Check sheet for the modelled part. Datum: model origin and axes. Units: mm. A direction names the side the tool comes from. Round coordinates to 2 decimals unless told otherwise and drop trailing zeros. Loops run counter-clockwise (first coordinate to the right, second up) from the corner with the lowest first, then second, coordinate; pieces in that order, holes last. Notation, with made-up numbers: (4, 84.5) -> (25, 84.5) arc R14 ccw to (25, 109.5) -> close; hole circle Ø11 at (1.25, 4). An arc over 180 degrees is marked (long way). Return JSON: item names as keys, results as strings.
Autodesk Inventor part; units mm, degrees
ref_plane "YZ Plane" through (0, 0, 0) normal (1, 0, 0) x (0, 1, 0)
ref_plane "XZ Plane" through (0, 0, 0) normal (0, 1, 0) x (-1, 0, 0)
ref_plane "XY Plane" through (0, 0, 0) normal (0, 0, 1) x (1, 0, 0)
sketch "Sketch5" plane through (0, 0, 0) normal (0, 1, 0) x (-1, 0, 0)
  circle A0 centre (177.8, -63.5) radius 3.9688
  circle A1 centre (50.8, -63.5) radius 3.9687
  line L0 (6.35, 0) -> (6.35, -6.35)
  line L1 (6.35, -6.35) -> (0, -6.35)
  line L2 (0, -6.35) -> (0, -12.7)
  line L3 (0, -12.7) -> (6.35, -12.7)
  line L4 (6.35, -12.7) -> (6.35, -19.05)
  line L5 (6.35, -19.05) -> (0, -19.05)
  line L6 (0, -19.05) -> (0, -25.4)
  line L7 (0, -25.4) -> (6.35, -25.4)
  line L8 (6.35, -25.4) -> (6.35, -31.75)
  line L9 (6.35, -31.75) -> (0, -31.75)
  line L10 (0, -31.75) -> (0, -38.1)
  line L11 (0, -38.1) -> (6.35, -38.1)
  line L12 (6.35, -38.1) -> (6.35, -44.45)
  line L13 (6.35, -44.45) -> (0, -44.45)
  line L14 (0, -44.45) -> (0, -50.8)
  line L15 (0, -50.8) -> (6.35, -50.8)
  line L16 (6.35, -50.8) -> (6.35, -57.15)
  line L17 (6.35, -57.15) -> (0, -57.15)
  line L18 (0, -57.15) -> (0, -63.5)
  line L19 (0, -63.5) -> (6.35, -63.5)
  line L20 (6.35, -63.5) -> (6.35, -69.85)
  line L21 (6.35, -69.85) -> (0, -69.85)
  line L22 (0, -69.85) -> (0, -76.2)
  line L23 (0, -76.2) -> (6.35, -76.2)
  line L24 (6.35, -76.2) -> (6.35, -82.55)
  line L25 (6.35, -82.55) -> (0, -82.55)
  line L26 (0, -82.55) -> (0, -88.9)
  line L27 (0, -88.9) -> (6.35, -88.9)
  line L28 (6.35, -88.9) -> (6.35, -95.25)
  line L29 (6.35, -95.25) -> (0, -95.25)
  line L30 (0, -95.25) -> (0, -101.6)
  line L31 (0, -101.6) -> (6.35, -101.6)
  line L32 (6.35, -101.6) -> (6.35, -107.95)
  line L33 (6.35, -107.95) -> (0, -107.95)
  line L34 (0, -107.95) -> (0, -114.3)
  line L35 (0, -114.3) -> (6.35, -114.3)
  line L36 (6.35, -114.3) -> (6.35, -120.65)
  line L37 (6.35, -120.65) -> (0, -120.65)
  line L38 (0, -120.65) -> (0, -127)
  line L39 (0, -127) -> (6.35, -127)
  line L40 (6.35, -127) -> (6.35, -133.35)
  line L41 (222.25, -133.35) -> (222.25, -127)
  line L42 (222.25, -127) -> (228.6, -127)
  line L43 (228.6, -127) -> (228.6, -120.65)
  line L44 (228.6, -120.65) -> (222.25, -120.65)
  line L45 (222.25, -120.65) -> (222.25, -114.3)
  line L46 (222.25, -114.3) -> (228.6, -114.3)
  line L47 (228.6, -114.3) -> (228.6, -107.95)
  line L48 (228.6, -107.95) -> (222.25, -107.95)
  line L49 (222.25, -107.95) -> (222.25, -101.6)
  line L50 (222.25, -101.6) -> (228.6, -101.6)
  line L51 (228.6, -101.6) -> (228.6, -95.25)
  line L52 (228.6, -95.25) -> (222.25, -95.25)
  line L53 (222.25, -95.25) -> (222.25, -88.9)
  line L54 (222.25, -88.9) -> (228.6, -88.9)
  line L55 (228.6, -88.9) -> (228.6, -82.55)
  line L56 (228.6, -82.55) -> (222.25, -82.55)
  line L57 (222.25, -82.55) -> (222.25, -76.2)
  line L58 (222.25, -76.2) -> (228.6, -76.2)
  line L59 (228.6, -76.2) -> (228.6, -69.85)
  line L60 (228.6, -69.85) -> (222.25, -69.85)
  line L61 (222.25, -69.85) -> (222.25, -63.5)
  line L62 (222.25, -63.5) -> (228.6, -63.5)
  line L63 (228.6, -63.5) -> (228.6, -57.15)
  line L64 (228.6, -57.15) -> (222.25, -57.15)
  line L65 (222.25, -57.15) -> (222.25, -50.8)
  line L66 (222.25, -50.8) -> (228.6, -50.8)
  line L67 (228.6, -50.8) -> (228.6, -44.45)
  line L68 (228.6, -44.45) -> (222.25, -44.45)
  line L69 (222.25, -44.45) -> (222.25, -38.1)
  line L70 (222.25, -38.1) -> (228.6, -38.1)
  line L71 (228.6, -38.1) -> (228.6, -31.75)
  line L72 (228.6, -31.75) -> (222.25, -31.75)
  line L73 (222.25, -31.75) -> (222.25, -25.4)
  line L74 (222.25, -25.4) -> (228.6, -25.4)
  line L75 (228.6, -25.4) -> (228.6, -19.05)
  line L76 (228.6, -19.05) -> (222.25, -19.05)
  line L77 (222.25, -19.05) -> (222.25, -12.7)
  line L78 (222.25, -12.7) -> (228.6, -12.7)
  line L79 (228.6, -12.7) -> (228.6, -6.35)
  line L80 (228.6, -6.35) -> (222.25, -6.35)
  line L81 (222.25, -6.35) -> (222.25, 0)
  line L82 (6.35, 0) -> (222.25, 0)
  line L83 (222.25, -133.35) -> (6.35, -133.35)
  point P0 (0, 0)
  dimension "Shaft_Diameter" = 7.9375
  dimension "d59" = 7.9375
  dimension "d73" = 6.35
  dimension "Teeth_Width" = 6.35
  dimension "d79" = 6.35
  dimension "d80" = 6.35
  dimension "d81" = 6.35
  dimension "d82" = 6.35
  dimension "d92" = 6.35
  dimension "d93" = 6.35
  dimension "d94" = 6.35
  dimension "d95" = 6.35
  dimension "d96" = 6.35
  dimension "d97" = 6.35
  dimension "d100" = 6.35
  dimension "d101" = 6.35
  dimension "d102" = 6.35
  dimension "d103" = 6.35
  dimension "d106" = 6.35
  dimension "d107" = 6.35
  dimension "d108" = 6.35
  dimension "d109" = 6.35
  dimension "d112" = 6.35
  dimension "d113" = 6.35
  dimension "d114" = 6.35
  dimension "d115" = 6.35
  dimension "d118" = 6.35
  dimension "d119" = 6.35
  dimension "d120" = 6.35
  dimension "d121" = 6.35
  dimension "d124" = 6.35
  dimension "d125" = 6.35
  dimension "d126" = 6.35
  dimension "d127" = 6.35
  dimension "d130" = 6.35
  dimension "d131" = 6.35
  dimension "d132" = 6.35
  dimension "d133" = 6.35
  dimension "d136" = 6.35
  dimension "d137" = 6.35
  dimension "d138" = 6.35
  dimension "d139" = 6.35
  dimension "d143" = 6.35
  dimension "d149" = 6.35
  dimension "d150" = 6.35
  dimension "d151" = 6.35
  dimension "d152" = 6.35
  dimension "d153" = 6.35
  dimension "d154" = 6.35
  dimension "d155" = 6.35
  dimension "d156" = 6.35
  dimension "d157" = 6.35
  dimension "d158" = 6.35
  dimension "d159" = 6.35
  dimension "d160" = 6.35
  dimension "d161" = 6.35
  dimension "d162" = 6.35
  dimension "d163" = 6.35
  dimension "d164" = 6.35
  dimension "d165" = 6.35
  dimension "d166" = 6.35
  dimension "d167" = 6.35
  dimension "d168" = 6.35
  dimension "d169" = 6.35
extrude "Extrusion4" add sketch "Sketch5" along normal blind 6.35
equation "\"d59\" = Shaft_Diameter"
properties part number "Base"
Q1. Tool access check on faces 1 (the flat face through (-6.35, 3, -130)), 2 (the flat face through (-3, 3, -19.05)), 3 (the flat face through (-225, 3, -63.5)), 4 (the flat face through (-228.6, 3, -124)), 5 (the flat face through (-222.25, 3, -130)). Record the directions out of +Z, -Z, +X, -X, +Y, -Y that give a thin tool (end or side, any length) a straight path to the whole face; none if there is none.
Results list:
{"face 1": "-Z, +X, +Y, -Y", "face 2": "+X, +Y, -Y", "face 3": "-X, +Y, -Y", "face 4": "+Z, -Z, -X, +Y, -Y", "face 5": "-Z, -X, +Y, -Y"}
Q2. Go/stop test with flat-tipped pins: pin 1 (1.9 mm diameter, centred on y = 2.5, z = -2.5, fed in from -X); pin 2 (1.9 mm diameter, centred on y = 2.5, z = -66, fed in from +X); pin 3 (3 mm diameter, centred on x = -224, y = 3.5, fed in from -Z). Record where each tip stops, or that it passes through.
Results list:
{"pin 1": "x = -222.25", "pin 2": "x = -6.35", "pin 3": "z = -127"}
Q3. Section check B-B (z = -40.5). Record the boundary of the cut face in (x, y), then the cut area to 3 significant figures.
Results list:
{"outline": "(-222.25, 0) -> (-6.35, 0) -> (-6.35, 6.35) -> (-222.25, 6.35) -> close", "area": "1,370 mm^2"}
Q4. Material ranges on line 1 (Z direction, x = -51, y = 2.5); line 2 (X direction, y = 5, z = -89), recorded low to high.
Results list:
{"line 1": "-133.35 to -67.46, -59.54 to 0", "line 2": "-222.25 to -6.35"}
Q5. Section check D-D (y = 4). Count the separate pieces of the cut face and the enclosed holes in it, then the cut area to 3 significant figures.
Results list:
{"separate pieces": "1", "enclosed holes": "2", "area": "29,500 mm^2"}
Q6. Draft check along Z on faces 6 (the flat face through (-116, 3, -133.35)), 7 (the flat face through (-225, 3, -82.55)), 8 (the flat face through (-228.6, 3, -10)). Enter one of: released by +Z, released by -Z, zero draft, split by the parting line, or undercut.
Results list:
{"face 6": "released by -Z", "face 7": "undercut", "face 8": "zero draft"}
Q7. Section check A-A (x = -177.8). Record the boundary of the cut face in (y, z).
Results list:
{"outline": "(0, -133.35) -> (6.35, -133.35) -> (6.35, -67.47) -> (0, -67.47) -> close; (0, -59.53) -> (6.35, -59.53) -> (6.35, 0) -> (0, 0) -> close"}
